Input: dimensioned drawing with shaded views. Units: mm. Origin: part minimum x, y, z. Coordinates: 2 decimals unless noted, no trailing zeros. Loops run counter-clockwise (first coordinate to the right, second up) from the corner with the lowest first, then second, coordinate; pieces in that order, holes last.
Item 1: Ray query, line 1 along Y through (x, z) = (57.5, 17.5); line 2 along Y through (x, z) = (78.5, 13.5); line 3 along Z through (x, y) = (67.5, 16.25). Return the intervals inside material, ascending.
Item 2: Section C-C on z = 6.25. Return loops of the section in (x, y), and give its area (3 significant figures).
Item 3: Section B-B on x = 65. Return loops of the section in (y, z) (1 decimal).
Item 4: Contact query for flat-ended pins moving along their axis: P1, Ø5, axis at x = 24, z = 9.5, coming from the +Y side; P2, Ø2, axis at y = 3, z = 9.5, coming from the -X side; P3, Ø8, axis at x = 76, z = 7.5, coming from the -Y side. Output: stop coordinate, or through.
Item 5: Section A-A on y = 1.5. Return loops of the section in (x, z).
Item 6: Pull-direction query (Z, two-part tool) for the marked faces 1, 2 and 3; classes: released by +Z, released by -Z, zero draft, split by the parting line, or undercut.
Item 7: Section D-D on y = 17. Return loops of the section in (x, z), and give its area (3 significant figures).
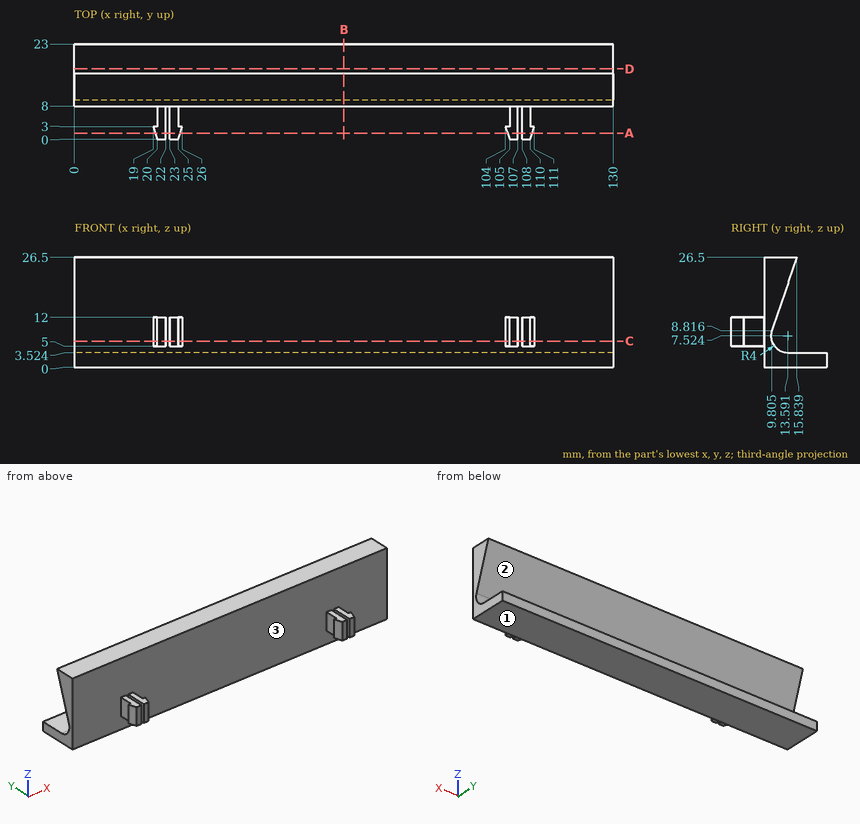
Results found:
1. line 1: y = 8 to 12.77
1. line 2: y = 8 to 11.4
1. line 3: z = 0 to 3.52
2. outline: (0, 8) - (20, 8) - (20, 3) - (19, 3) - (20, 0) - (22, 0) - (22, 8) - (23, 8) - (23, 0) - (25, 0) - (26, 3) - (25, 3) - (25, 8) - (105, 8) - (105, 3) - (104, 3) - (105, 0) - (107, 0) - (107, 8) - (108, 8) - (108, 0) - (110, 0) - (111, 3) - (110, 3) - (110, 8) - (130, 8) - (130, 9.8) - (0, 9.8) - close
2. area: 304 mm2
3. outline: (8, 0) - (23, 0) - (23, 3.5) - (13.6, 3.5) arc R4 cw to (9.8, 8.8) - (15.8, 26.5) - (8, 26.5) - close
4. P1: stops at y = 10.89
4. P2: stops at x = 19
4. P3: stops at y = 8
5. outline: (19.5, 5) - (22, 5) - (22, 12) - (19.5, 12) - close; (23, 5) - (25.5, 5) - (25.5, 12) - (23, 12) - close; (104.5, 5) - (107, 5) - (107, 12) - (104.5, 12) - close; (108, 5) - (110.5, 5) - (110.5, 12) - (108, 12) - close
6. face 1: released by -Z
6. face 2: undercut
6. face 3: zero draft
7. outline: (0, 0) - (130, 0) - (130, 3.52) - (0, 3.52) - close
7. area: 458 mm2
